The model under review builds one solid part; all positions refer to its coordinate system, in mm. Face numbers are marked on the shaded views. A direction names the side the tool comes from. Coordinates: 2 decimals unless noted, no trailing zeros. Loops run counter-clockwise (first coordinate to the right, second up) from the corner with the lowest first, then second, coordinate; pieces in that order, holes last. Notation, with made-up numbers: M 61,19 L 111,19 A20 cw 111,40 Z; hole C -26,-10 d9. An arc over 180 degrees is marked long. Use CSV: the item, a comma, the result in double quotes. Start each with the question number.
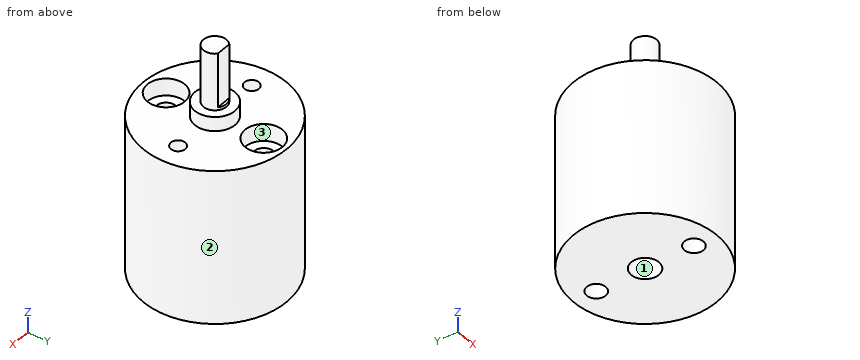
from build123d import *

# Parameters (mm, degrees)
F0_R           = 12.5
F1_DEPTH       = 27
F2_R           = 3.5
F3_DEPTH       = 2.5
F4_R           = 2
F5_DEPTH       = 10
F7_D           = 2.5
F7_DEPTH       = 8.5
F7_TIP         = 0.7510757738
F8_D           = 3.3
F8_CBORE_D     = 6.5
F8_CBORE_DEPTH = 3
F9_R           = 2.4
F10_DEPTH      = 6.5
F11_W          = 2.6457513111
F11_H          = 0.5
F12_DEPTH      = 9.5


with BuildPart() as f1:
    # F0 (on Top) → F1 (new body)
    with BuildSketch(Plane.XY):
        Circle(F0_R)
    extrude(amount=F1_DEPTH)

    # F2 (on face) → F3 (join)
    with BuildSketch(Plane.XY.offset(27)):
        Circle(F2_R)
    extrude(amount=F3_DEPTH)

    # F4 (on face) → F5 (join)
    with BuildSketch(Plane.XY.offset(29.5)):
        Circle(F4_R)
    extrude(amount=F5_DEPTH)

    # F7
    with Locations(Plane.XY.offset(27)):
        with Locations((-8.5, 0), (8.5, 0)):
            Hole(F7_D / 2, depth=F7_DEPTH)
            with Locations((0, 0, -(F7_DEPTH + F7_TIP / 2))):  # 118° drill point
                Cone(0, F7_D / 2, F7_TIP, mode=Mode.SUBTRACT)

    # F8 (through all)
    with Locations(Plane.XY.offset(27)):
        with Locations((0, 8.5), (0, -8.5)):
            CounterBoreHole(F8_D / 2, F8_CBORE_D / 2, F8_CBORE_DEPTH)

    # F9 (on face) → F10 (cut)
    with BuildSketch(Plane(origin=(0, 0, 0), x_dir=(1, 0, 0), z_dir=(0, 0, -1))):
        Circle(F9_R)
    extrude(amount=-F10_DEPTH, mode=Mode.SUBTRACT)

    # F11 (on face) → F12 (cut)
    with BuildSketch(Plane.XY.offset(39.5)):
        with Locations((0, 1.75)):
            Rectangle(F11_W, F11_H)
    extrude(amount=-F12_DEPTH, mode=Mode.SUBTRACT)


solid = f1.part
1. Add section A-A (x = 0). Give the number of separate pieces and of enclosed holes in the cut face, plus the area to 3 significant figures.
2. Insertion check: pin 1 Ø7 at (x, y) = (-0.5, 7.5) entering from +Z; pin 2 Ø3 at (x, y) = (1, -9.5) entering from +Z; pin 3 Ø1.5 at (x, y) = (-9, -10) entering from -Z; pin 4 Ø1.3 at (x, z) = (0, 33.5) entering from +Y. Each pin has a flat end and moves straight along its axis. Give the tip position at first contact, or say it passes through.
3. For the marked faces 1, 2 and 3, list the 3-axis set-ups (+Z, -Z, +X, -X, +Y, -Y) from which the entire face can be reached by the end or side of a thin tool; tool diameter is ignored.
4. To check wall thickness, follow line 1 along Y through (x, z) = (0, 26.2); line 2 along Y through (x, z) = (0, 11.75); line 3 along Z through (x, y) = (3.5, -9.5). State the ranges of each line that lie inside material, in increasing order.
5. Add section B-B (z = 21). Write out the cut boundary in (x, y).
6. Add section D-D (z = 13). Write out the cut boundary in (x, y).
7. Add section C-C (y = -8.5). Write out the cut boundary in (x, z).
Solved:
1,separate pieces,"3"
1,enclosed holes,"0"
1,area,"499 mm^2"
2,pin 1,"stops at z = 27"
2,pin 2,"stops at z = 24"
2,pin 3,"passes through"
2,pin 4,"stops at y = 1.5"
3,face 1,"-Z"
3,face 2,"+Z, -Z"
3,face 3,"+Z"
4,line 1,"y = -12.5 to -11.75, -5.25 to 5.25, 11.75 to 12.5"
4,line 2,"y = -12.5 to -10.15, -6.85 to 6.85, 10.15 to 12.5"
4,line 3,"z = 0 to 27"
5,outline,"C 0,0 d25; hole C -8.5,0 d2.5; hole C 0,-8.5 d3.3; hole C 0,8.5 d3.3; hole C 8.5,0 d2.5"
6,outline,"C 0,0 d25; hole C 0,-8.5 d3.3; hole C 0,8.5 d3.3"
7,outline,"M -9.17,0 L -1.65,0 L -1.65,24 L -3.25,24 L -3.25,27 L -9.17,27 Z; M 1.65,0 L 9.17,0 L 9.17,27 L 3.25,27 L 3.25,24 L 1.65,24 Z"
